The drawing under review shows one solid part. Ordinate dimensions are in mm from its lowest x, y, z. Round coordinates to 2 decimals unless told otherwise and drop trailing zeros. Order: outer loops, then holes, each group sorted by start corner. A loop starts at its lowest first (then second) coordinate and runs counter-clockwise, first axis right, second up.
1) Consider section A-A (x = 47.5). Give the boundary of the cut face in (y, z) (1 decimal).
2) Consider section B-B (x = 25). Give the boundary of the cut face in (y, z) (1 decimal).
3) Consider section C-C (x = 33.5). Give the boundary of the cut face in (y, z) (1 decimal).
4) To check wall thickness, follow L1, parallel to Z at x = 49, y = 1.3; L2, parallel to Z at x = 47, y = 1.95 (1 decimal); L3, parallel to X at y = 2.3, z = 19 (1 decimal). State the ranges of each line that lie inside material, in increasing order.
5) Clearance check with flat-ended pins moving along their axes: P1, Ø6, axis at x = 30, z = 37, coming from the -Y side; P2, Ø1, axis at x = 40, y = 1.5, coming from the +Z side; P3, Ø1.2, axis at y = 1, z = 35.5, coming from the -X side (1 decimal); P4, Ø1.2, axis at y = 2, z = 35, coming from the +X side (1 decimal). State where each tip first meets the part, or that it passes through.
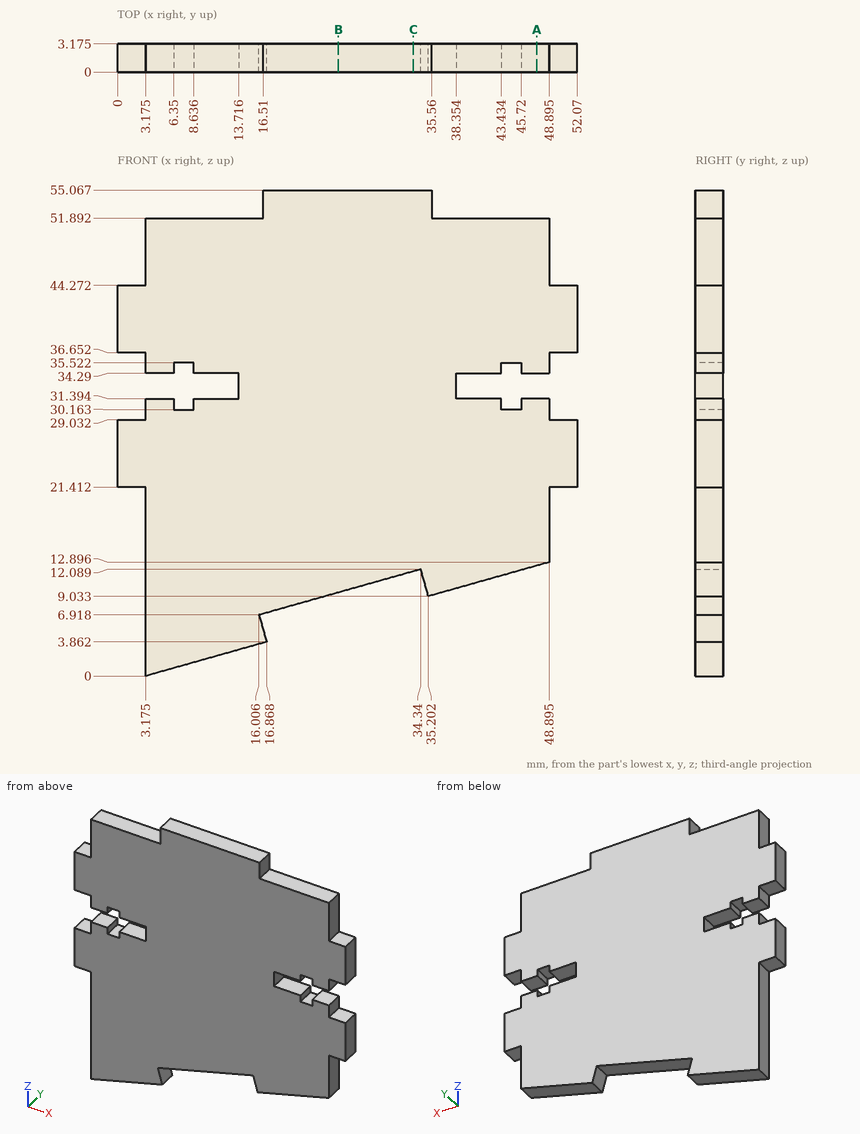
Answer below:
1. outline: (0, 12.5) - (3.2, 12.5) - (3.2, 31.4) - (0, 31.4) - close; (0, 34.3) - (3.2, 34.3) - (3.2, 51.9) - (0, 51.9) - close
2. outline: (0, 9.5) - (3.2, 9.5) - (3.2, 55.1) - (0, 55.1) - close
3. outline: (0, 11.9) - (3.2, 11.9) - (3.2, 55.1) - (0, 55.1) - close
4. L1: z = 21.41 to 29.03, 36.65 to 44.27
4. L2: z = 12.4 to 31.4, 34.3 to 51.9
4. L3: x = 3.2 to 48.9
5. P1: stops at y = 0
5. P2: stops at z = 51.89
5. P3: stops at x = 3.2
5. P4: stops at x = 48.9
